Design review of the part built by this model. Coordinates are the model's own, in mm. Coordinates: 2 decimals unless noted, no trailing zeros. Write each loop counter-clockwise with the first axis right and the second up, starting at its lowest first coordinate (ties: lowest second). Pieces come first, ordered by that corner, then holes. Notation, with made-up numbers: (-11, 48) - (27, 48) arc R28 ccw to (27, 75) - close; hole circle Ø10 at (-21, -14). An arc over 180 degrees is marked (long way). Answer as CSV lines item,"result". Start each with the question number.
Q1. For line 1 along Y through (x, z) = (2.5, 0.65); line 2 along Y through (x, z) = (0.25, 0.2); line 3 along Y through (x, z) = (-2.25, 0.45), list the stretches that pass through material, from the lowest coordinate up. Write a range as [from, to].
Q2. We need section C-C (y = 9.5). Write out the cut boundary in (x, z), plus the area to 3 significant figures.
Q3. We need section A-A (z = 1.55). Write out the cut boundary in (x, y), plus the area to 3 significant figures.
Q4. We need section B-B (y = 52). Write out the cut boundary in (x, z), plus the area to 3 significant figures.
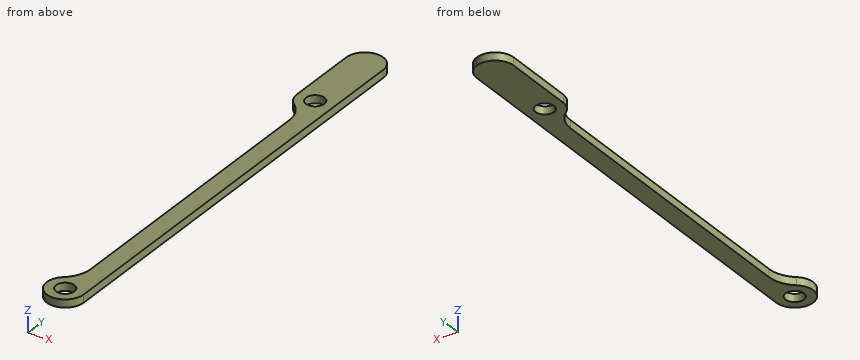
from build123d import *

# Parameters (mm, degrees)
MODEL_R             = 3
BOSS_EXTRUDE1_DEPTH = 2.55


with BuildPart() as part:
    # Model → Boss-Extrude1 (new body)
    with BuildSketch(Plane.XY):
        with BuildLine():
            Line((6, 120), (6, 145))
            ThreePointArc((6, 145), (0, 151), (-6, 145))
            Line((-6, 145), (-6, 121))
            ThreePointArc((-6, 121), (-5.408326913, 118.401923789), (-3.75, 116.316251501))
            ThreePointArc((-3.75, 116.316251501), (-0.986121811, 112.840131022), (0, 108.510004003))
            Line((0, 108.510004003), (0, 12.489995997))
            ThreePointArc((0, 12.489995997), (-0.986121811, 8.159868978), (-3.75, 4.683748499))
            ThreePointArc((-3.75, 4.683748499), (-2.598076211, -5.408326913), (6, 0))
            Line((6, 0), (6, 120))
        make_face()
        Circle(MODEL_R, mode=Mode.SUBTRACT)
        with Locations((0, 121)):
            Circle(MODEL_R, mode=Mode.SUBTRACT)
    extrude(amount=BOSS_EXTRUDE1_DEPTH)


solid = part.part
Results list:
1,line 1,"y = [-5.45, -1.66], [1.66, 119.34], [122.66, 150.45]"
1,line 2,"y = [-5.99, -2.99], [2.99, 118.01], [123.99, 150.99]"
1,line 3,"y = [-5.56, -1.98], [1.98, 6.17], [114.83, 119.02], [122.98, 150.56]"
2,outline,"(-0.46, 0) - (6, 0) - (6, 2.55) - (-0.46, 2.55) - close"
2,area,"16.5 mm2"
3,outline,"(-6, 121) arc R6 ccw to (-3.75, 116.32) arc R10 cw to (0, 108.51) - (0, 12.49) arc R10 cw to (-3.75, 4.68) arc R6 ccw (long way) to (6, 0) - (6, 145) arc R6 ccw to (-6, 145) - close; hole circle Ø6 at (0, 0); hole circle Ø6 at (0, 121)"
3,area,"1,140 mm2"
4,outline,"(0, 0) - (6, 0) - (6, 2.55) - (0, 2.55) - close"
4,area,"15.3 mm2"
